Here's how the part is built. I have some questions about the finished solid (model axes, mm). A direction names the side the tool comes from. Coordinates: 2 decimals unless noted, no trailing zeros. Write each loop counter-clockwise with the first axis right and the second up, starting at its lowest first coordinate (ties: lowest second). Pieces come first, ordered by that corner, then holes.
Item 1: I want a section at D-D (y = 47.5). Please give me the cut outline in (x, z).
Item 2: Please list where these lines run through material, in increasing order: line 1 (Z direction, x = 4, y = 59); line 2 (X direction, y = 28.5, z = 60.5); line 3 (Y direction, x = 29.5, z = 74).
Item 3: I want a section at B-B (x = 46). Please give me the cut outline in (y, z), and give its area (3 significant figures).
Item 4: For faces 5 (the face through (62, 45, 0)), 6 (the face through (33.624, 29, 16)), 7 (the face through (32, 10, 33)), 8 (the face through (56.66, 54.5, -6.08)), which set-ups out of +Z, -Z, +X, -X, +Y, -Y let a thin tool reach every point of the face, with its end or its side?
Item 5: I'm going to push flat-ended pins straight in: P1, Ø11, axis at x = 61, y = 40.5, coming from the +Z side; P2, Ø20.5, axis at y = 42.5, z = 17, coming from the +X side; P3, Ø12, axis at x = 21.5, z = 11.5, coming from the +Y side. Where does each tip first touch, or does it pass through?
Item 6: I want a section at A-A (y = 58.5). Please give me the cut outline in (x, z), and give its area (3 significant figures).
Item 7: I want a section at C-C (y = 16.5). Please give me the cut outline in (x, z).
Item 8: If we mould it in two halves opening along Z, with no side actions, what happens to faces 1 (the face through (41.516, 5.07, 85.833)), 2 (the face through (75.72, 75.49, -6.08)), 3 (the face through (32.7, 24.8, 63.2)), 4 (the face through (43.624, 29, 16))? For each: pulls with the +Z half, pulls with the -Z half, needs draft (parallel to the pull), parting line crosses it, or undercut.
from build123d import *

# Parameters (mm, degrees)
BOSS_EXTRUDE2_DEPTH      = 10
CUT_EXTRUDE_THIN1_DEPTH  = 10
SKETCH5_R                = 17.5
SKETCH5_R_2              = 10
BOSS_EXTRUDE3_DEPTH      = 30
SKETCH7_W                = 80
SKETCH7_H                = 80
BOSS_EXTRUDE4_DEPTH      = 12
FILLET2_R                = 15
BOSS_EXTRUDE5_REACH      = 144.014
BOSS_EXTRUDE5_END_RADIUS = 17.5
SKETCH8_W                = 10
SKETCH8_H                = 70
SKETCH9_R                = 39.5
CUT_EXTRUDE1_DEPTH       = 12
F_10_0MM_DOWEL_SLOT1_D   = 10


with BuildPart() as part:
    # Sketch3 → Boss-Extrude2 (new body)
    with BuildSketch(Plane(origin=(0, 0, 0), x_dir=(1, 0, 0), z_dir=(0, 1, 0))):
        with BuildLine():
            Line((0, 0), (80, 0))
            add(Edge.make_bspline(
                [(0, 0), (9.568772754, -3.662252769), (13.233792617, -26.367514399), (14.892974138, -48.26173719), (19.457625693, -73.382546531), (29.234028115, -88.842620539), (47.339429681, -94.978505807), (65.072681899, -76.355870434), (65.472290622, -49.499797191), (60.330152399, -17.820535728), (73.673313223, -1.004614773), (80, 0)],
                knots=[0, 0, 0, 0, 0.130431735, 0.366934607, 0.413509275, 0.549603742, 0.580090258, 0.687887922, 0.718701469, 0.85741218, 1, 1, 1, 1], degree=3))
        make_face()
    extrude(amount=BOSS_EXTRUDE2_DEPTH)

    # Sketch4 → Cut-Extrude-Thin1 (cut)
    with BuildSketch(Plane(origin=(0, 10, 0), x_dir=(1, 0, 0), z_dir=(0, 1, 0))):
        Polygon((7.236393203, -67.338737313), (6.633563606, -66.218935394), (15.43873628, -61.47879466), (16.041565876, -62.598596579), align=None)
        with BuildLine():
            ThreePointArc((20.05548635, -71.393733338), (41.904058586, -85.836536546), (63.752630822, -71.393733338))
            Line((63.752630822, -71.393733338), (72.953082149, -75.311857301))
            ThreePointArc((72.953082149, -75.311857301), (41.904058586, -95.836536546), (10.855035023, -75.311857301))
            Line((10.855035023, -75.311857301), (20.05548635, -71.393733338))
        make_face()
    extrude(amount=-CUT_EXTRUDE_THIN1_DEPTH, mode=Mode.SUBTRACT)

    # Sketch5 → Boss-Extrude3 (add)
    with BuildSketch(Plane(origin=(0, 10, 0), x_dir=(1, 0, 0), z_dir=(0, 1, 0))):
        with Locations(Location((41.563187494, -58.566374958, 0), (0, 0, 270))):
            Circle(SKETCH5_R)
        with Locations(Location((41.563187494, -58.566374958, 0), (0, 0, 270))):
            Circle(SKETCH5_R_2, mode=Mode.SUBTRACT)
    extrude(amount=BOSS_EXTRUDE3_DEPTH)

    # Sketch7 → Boss-Extrude4 (add)
    with BuildSketch(Plane(origin=(0, 0, 0), x_dir=(-1, 0, 0), z_dir=(0, 0, -1))):
        with Locations((-40, 40)):
            Rectangle(SKETCH7_W, SKETCH7_H)
    extrude(amount=BOSS_EXTRUDE4_DEPTH)

    # Fillet2
    fillet2_edges = [part.edges().sort_by_distance(p)[0] for p in [
        (80, 80, -6),
        (0, 80, -6),
    ]]
    fillet(fillet2_edges, radius=FILLET2_R)

    # Boss-Extrude5: up to this cylinder (the profile starts outside it)
    boss_extrude5_end = Plane(origin=(41.563187494, 45, 58.566374958), z_dir=(0, -1, 0)) * Cylinder(BOSS_EXTRUDE5_END_RADIUS, 324.028, mode=Mode.PRIVATE)
    # Sketch8 → Boss-Extrude5 (add, up to the surface)
    with BuildSketch(Plane.XY, mode=Mode.PRIVATE) as boss_extrude5_sk1:
        with Locations((38.624100389, 45)):
            Rectangle(SKETCH8_W, SKETCH8_H)
    boss_extrude5_tool1 = extrude(boss_extrude5_sk1.sketch, amount=BOSS_EXTRUDE5_REACH, mode=Mode.PRIVATE) - boss_extrude5_end
    add(boss_extrude5_tool1.solids().sort_by_distance((38.6241, 45, 0))[0])

    # Sketch9 → Cut-Extrude1 (cut)
    with BuildSketch(Plane.ZY.offset(-33.624100389)):
        with Locations((39.952210093, 80)):
            Circle(SKETCH9_R)
    extrude(amount=-CUT_EXTRUDE1_DEPTH, mode=Mode.SUBTRACT)

    # Ø10.0mm Dowel Slot1 (through all)
    with Locations(Plane.XY):
        with Locations((61.279203802, 56.41280999), (16.414291642, 56.41280999)):
            Hole(F_10_0MM_DOWEL_SLOT1_D / 2)


solid = part.part
Answer:
1. outline: (0, -12) - (80, -12) - (80, 0) - (43.62, 0) - (43.62, 17.5) - (33.62, 17.5) - (33.62, 0) - (0, 0) - close
2. line 1: z = -12 to 0
2. line 2: x = 24.17 to 31.75, 51.37 to 58.96
2. line 3: y = 0 to 10
3. outline: (0, -12) - (80, -12) - (80, 0) - (10, 0) - (10, 41.64) - (40, 41.64) - (40, 49.6) - (10, 49.6) - (10, 67.53) - (40, 67.53) - (40, 75.49) - (10, 75.49) - (10, 85.48) - (0, 85.48) - close
3. area: 2,290 mm2
4. face 5: +X, +Y
4. face 6: -X, +Y
4. face 7: +Y
4. face 8: +Z, -Z
5. P1: stops at z = 69.12
5. P2: stops at x = 43.62
5. P3: stops at y = 10
6. outline: (0, -12) - (11.87, -12) - (11.87, 0) - (0, 0) - close; (20.96, -12) - (56.74, -12) - (56.74, 0) - (43.62, 0) - (43.62, 6.82) - (33.62, 6.82) - (33.62, 0) - (20.96, 0) - close; (65.82, -12) - (80, -12) - (80, 0) - (65.82, 0) - close
6. area: 810 mm2
7. outline: (0, -12) - (80, -12) - (80, 0) - (43.62, 0) - (43.62, 41.19) arc R17.5 ccw (long way) to (33.62, 42.97) - (33.62, 0) - (0, 0) - close; hole circle Ø20 at (41.56, 58.57)
8. face 1: pulls with the +Z half
8. face 2: needs draft
8. face 3: undercut
8. face 4: undercut
